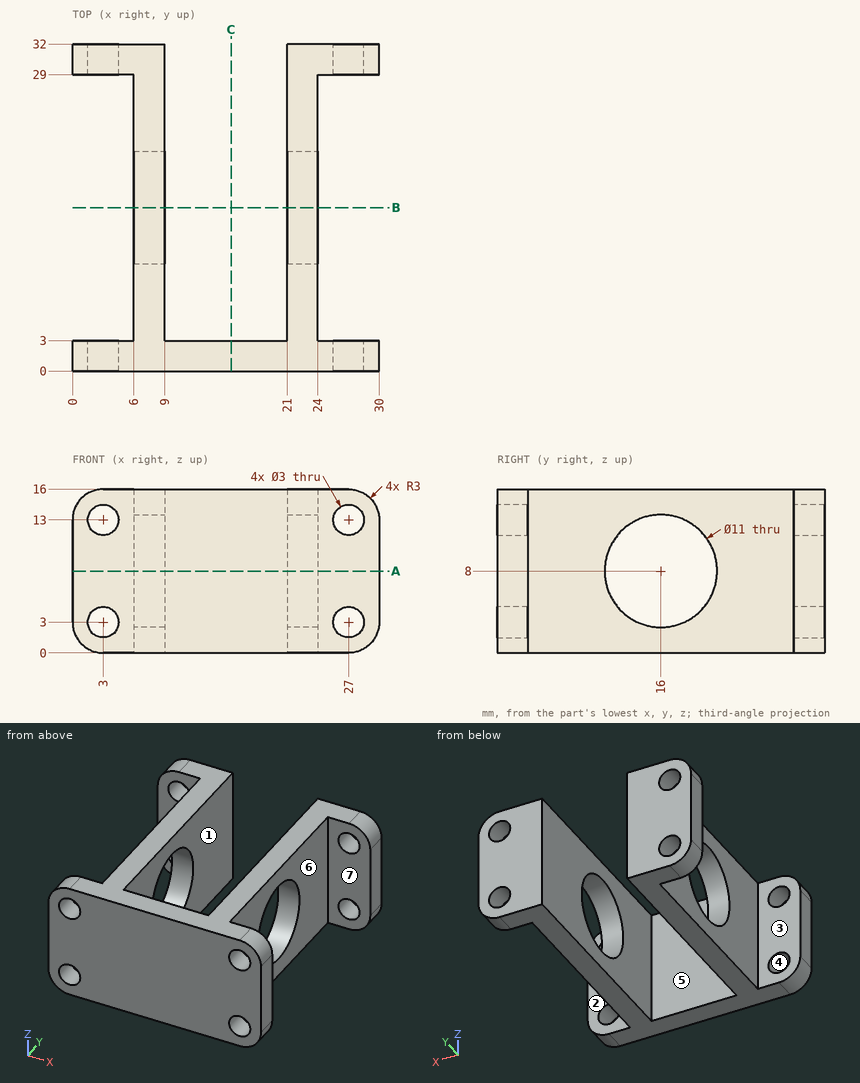
Input: dimensioned drawing with shaded views. Units: mm. Origin: part minimum x, y, z. A direction names the side the tool comes from. Round coordinates to 2 decimals unless told otherwise and drop trailing zeros. Order: outer loops, then holes, each group sorted by start corner. A loop starts at its lowest first (then second) coordinate and runs counter-clockwise, first axis right, second up. Notation, with made-up numbers: (48, 63) -> (89, 63) arc R9 cw to (89, 76) -> close; hole circle Ø2 at (-6.75, -11.5). An arc over 180 degrees is marked (long way). One line per item, written item: value. Start each with the question number.
Q1. Access query for the marked faces 1, 2 and 3. Directions: +Z, -Z, +X, -X, +Y, -Y. A direction counts if a zero-diameter tool reaches every point of the face in a straight line with its end or side. Return the directions, or none.
Q2. Draft query along Y for the marked faces 4, 5, 6 and 7. Return one class per face: pulls with the +Y half, pulls with the -Y half, needs draft (parallel to the pull), parting line crosses it, or undercut.
Q3. Section query A-A (z = 8). Return the cut outline in (x, y), plus the area to 3 significant figures.
Q4. Section query C-C (x = 15.5). Return the cut outline in (y, z).
Q5. Pin query (flat end, axial travel): pin 1 (3 mm diameter, centred on y = 19, z = 10.5, fed in from -X); pin 2 (6 mm diameter, centred on y = 20, z = 11.5, fed in from +X); pin 3 (5 mm diameter, centred on y = 11.5, z = 6.5, fed in from -X); pin 4 (9.5 mm diameter, centred on x = 15.5, z = 10, fed in from +Y). Return the tip coordinate at first contact, or that it passes through.
Q6. Section query B-B (y = 16). Return the cut outline in (x, z), plus the area to 3 significant figures.
Q7. Material intervals for probe 1 along X at (y, z) = (30.3, 13); probe 2 along X at (y, z) = (2.1, 13); probe 3 along X at (y, z) = (23.5, 11), sorted ascending.
Findings below:
1. face 1: +Z, -Z, +Y
1. face 2: +Z, -Z, +X
1. face 3: +Z, -Z, -X
2. face 4: needs draft
2. face 5: pulls with the +Y half
2. face 6: undercut
2. face 7: undercut
3. outline: (0, 0) -> (30, 0) -> (30, 3) -> (24, 3) -> (24, 10.5) -> (21, 10.5) -> (21, 3) -> (9, 3) -> (9, 10.5) -> (6, 10.5) -> (6, 3) -> (0, 3) -> close; (0, 29) -> (6, 29) -> (6, 21.5) -> (9, 21.5) -> (9, 32) -> (0, 32) -> close; (21, 21.5) -> (24, 21.5) -> (24, 29) -> (30, 29) -> (30, 32) -> (21, 32) -> close
3. area: 234 mm²
4. outline: (0, 0) -> (3, 0) -> (3, 16) -> (0, 16) -> close
5. pin 1: through
5. pin 2: x = 24
5. pin 3: x = 6
5. pin 4: y = 3
6. outline: (6, 0) -> (9, 0) -> (9, 2.5) -> (6, 2.5) -> close; (6, 13.5) -> (9, 13.5) -> (9, 16) -> (6, 16) -> close; (21, 0) -> (24, 0) -> (24, 2.5) -> (21, 2.5) -> close; (21, 13.5) -> (24, 13.5) -> (24, 16) -> (21, 16) -> close
6. area: 30.0 mm²
7. probe 1: 0 to 1.5, 4.5 to 9, 21 to 25.5, 28.5 to 30
7. probe 2: 0 to 1.5, 4.5 to 25.5, 28.5 to 30
7. probe 3: 6 to 9, 21 to 24
